For this review, take the finished solid that the model builds, in its own axes (mm). Face numbers are marked on the shaded views. Give positions to 0.01 mm unless a question says otherwise; leave off trailing zeros. Return JSON: item names as keys, results as strings. Group by question number.
1) Insertion check: P1, Ø1.5, axis at y = 20, z = 14.5, coming from the -X side; P2, Ø2, axis at x = 18, z = 12.5, coming from the -Y side; P3, Ø6, axis at x = 26.5, z = 21, coming from the +Y side. Each pin has a flat end and moves straight along its axis. Give the tip position at first contact, or say it passes through.
2) The part is to be moulded in two halves that separate along Y. For the marked faces 1 and 2, say which applies: released by +Y, released by -Y, zero draft, split by the parting line, or undercut.
3) To check wall thickness, follow line 1 along X through (y, z) = (13.5, 7.5); line 2 along X through (y, z) = (13.5, 24); line 3 along Y through (x, z) = (13.5, 11.5). State the ranges of each line that lie inside material, in increasing order.
from build123d import *

# Parameters (mm, degrees)
PAD_DEPTH = 30
BOX_W     = 10
BOX_H     = 10
BOX_DEPTH = 10


with BuildPart() as part:
    # Sketch (on XY_Plane of Origin) → Pad (new body)
    with BuildSketch(Plane.XY):
        with BuildLine():
            ThreePointArc((25.9, 8e-06), (18.314063, 18.314069), (0, 25.9))
            Line((0, 25.9), (0, 30.9))
            Line((0, 30.9), (0, 30.98))
            ThreePointArc((30.98, 0), (21.906168, 21.906168), (0, 30.98))
            Line((30.9, 0), (30.98, 0))
            Line((25.9, 8e-06), (30.9, 0))
        make_face()
    extrude(amount=PAD_DEPTH)

    # Box → Box (cut)
    with BuildSketch(Plane.XY):
        with Locations((5, 5)):
            Rectangle(BOX_W, BOX_H)
    extrude(amount=BOX_DEPTH, mode=Mode.SUBTRACT)

    # Sketch001 (on XZ_Plane of Origin) → Groove (revolve, cut)
    with BuildSketch(Plane.XZ):
        with BuildLine():
            ThreePointArc((25.828939, 0), (29.840979, 14.944895), (25.828939, 29.88979))
            Line((25.828939, 29.88979), (25.828939, 0))
        make_face()
    revolve(axis=Axis((0, 0, 0), (0, 0, 1)), mode=Mode.SUBTRACT)


solid = part.part
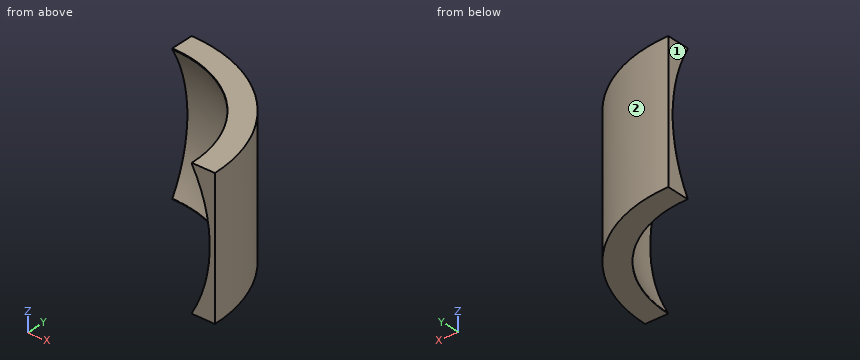
Evaluation:
{
 "1": {"P1": "x = 21.44", "P2": "y = 22.87", "P3": "y = 20.19"},
 "2": {"face 1": "zero draft", "face 2": "released by +Y"},
 "3": {"line 1": "25.55 to 27.88", "line 2": "25.02 to 27.88", "line 3": "26.39 to 27.88"}
}
